The model under review builds one solid part; all positions refer to its coordinate system, in mm. A direction names the side the tool comes from. Give positions to 0.01 mm unless a question says otherwise; leave off trailing zeros. Order: outer loops, then holes, each group sorted by start corner. A loop starts at its lowest first (then second) coordinate and runs counter-clockwise, first axis right, second up. Notation, with made-up numbers: M 37.25,36 L 86.25,36 A15 cw 86.25,50 Z; hole C 79.25,32 d2. An arc over 180 degrees is marked long. One line per question, with ' | ' between items. Start each with the question number.
1. Wall thickness on L1, parallel to Y at x = 0, z = -8.95; L2, parallel to X at y = 5.25, z = 2; L3, parallel to X at y = 2.25, z = 5.75: over which ranges is each line inside the solid? List them lowest first.
2. For faces 1 (the face through (-2.2, -10, -9.5)), 2 (the face through (3, 3, 1)), 3 (the face through (0, -7, -8.5)), list the 3-axis set-ups (+Z, -Z, +X, -X, +Y, -Y) from which the entire face can be reached by the end or side of a thin tool; tool diameter is ignored.
3. We need section B-B on y = -10. Write out the cut boundary in (x, z).
4. Insertion check: P1, Ø3.5, axis at x = 0, y = -10, coming from the -Z side; P2, Ø1, axis at x = -0.5, y = -2, coming from the +Z side; P3, Ø8, axis at y = -9.5, z = -2, coming from the +X side; P4, Ø2.5, axis at x = -0.5, z = 7.5, coming from the -Y side. Each pin has a flat end and moves straight along its axis. Give the tip position at first contact, or say it passes through.
5. We need section A-A on x = 0. Write out the cut boundary in (y, z), then the cut area to 3 significant figures.
6. The part is to be moulded in two halves that separate along X. For faces 4 (the face through (0, 3, -2.5)), 5 (the face through (-5.18, -19.4, -10.48)), 6 (the face through (0, 0, -5)), 7 (the face through (-3, 3, 1)), say which applies: +X half, -X half, draft (parallel to the pull), parting line (faces both ways), or undercut.
7. We need section C-C on z = -6. Write out the cut boundary in (x, y), then the cut area to 3 significant figures.
8. We need section D-D on y = 3.75. Write out the cut boundary in (x, z), then the cut area to 3 significant figures.
```python
from build123d import *

# Parameters (mm, degrees)
SKETCH1_W                      = 11.5
SKETCH1_H                      = 25
BOSS_EXTRUDE1_DEPTH            = 8
CUT_EXTRUDE1_DEPTH             = 6
SKETCH3_W                      = 11.5
SKETCH3_H                      = 4
BOSS_EXTRUDE2_DEPTH            = 20
CBORE_FOR_M3_SHCS1_D           = 3.2
CBORE_FOR_M3_SHCS1_CBORE_D     = 6.6
CBORE_FOR_M3_SHCS1_CBORE_DEPTH = 3
FILLET1_R                      = 2
CHAMFER1_SIZE                  = 0.4
CHAMFER2_SIZE                  = 0.4


with BuildPart() as part:
    # Sketch1 → Boss-Extrude1 (new body)
    with BuildSketch(Plane(origin=(0, 0, 0), x_dir=(1, 0, 0), z_dir=(0, 1, 0))):
        Rectangle(SKETCH1_W, SKETCH1_H)
    extrude(amount=BOSS_EXTRUDE1_DEPTH)

    # Sketch2 → Cut-Extrude1 (cut)
    with BuildSketch(Plane.XZ):
        Polygon((-3, 12.5), (3, 12.5), (3, 11.5), (3.8, 11.5), (3.8, 4.5), (3, 4.5), (3, -2.5), (-3, -2.5), (-3, 4.5), (-3.8, 4.5), (-3.8, 11.5), (-3, 11.5), align=None)
    extrude(amount=-CUT_EXTRUDE1_DEPTH, mode=Mode.SUBTRACT)

    # Sketch3 → Boss-Extrude2 (add)
    with BuildSketch(Plane.XZ):
        with Locations((0, -10.5)):
            Rectangle(SKETCH3_W, SKETCH3_H)
    extrude(amount=BOSS_EXTRUDE2_DEPTH)

    # CBORE for M3 SHCS1 (through all)
    with Locations(Plane(origin=(0, 0, -12.5), x_dir=(-1, 0, 0), z_dir=(0, 0, -1))):
        with Locations((0, -10)):
            CounterBoreHole(CBORE_FOR_M3_SHCS1_D / 2, CBORE_FOR_M3_SHCS1_CBORE_D / 2, CBORE_FOR_M3_SHCS1_CBORE_DEPTH)

    # Fillet1
    fillet1_edges = [part.edges().sort_by_distance(p)[0] for p in [
        (-5.75, -20, -10.5),
        (5.75, -20, -10.5),
    ]]
    fillet(fillet1_edges, radius=FILLET1_R)

    # Chamfer1
    chamfer1_edges = [part.edges().sort_by_distance(p)[0] for p in [
        (5.75, 8, 0),
        (0, 8, -12.5),
        (-5.75, 8, 0),
        (0, 8, 12.5),
    ]]
    chamfer(chamfer1_edges, length=CHAMFER1_SIZE)

    # Chamfer2
    chamfer2_edges = [part.edges().sort_by_distance(p)[0] for p in [
        (4.375, 0, 12.5),
        (-3, 0, 12),
        (-3.4, 0, 11.5),
        (-3.8, 0, 8),
        (-3.4, 0, 4.5),
        (-3, 0, 1),
        (0, 0, -2.5),
        (3, 0, 1),
        (3.4, 0, 4.5),
        (3.8, 0, 8),
        (3.4, 0, 11.5),
        (3, 0, 12),
        (3, 3, 12.5),
        (0, 6, 12.5),
        (-3, 3, 12.5),
        (-5.75, 0, 2),
        (5.75, 0, 2),
        (-4.375, 0, 12.5),
        (3.3, -10, -12.5),
        (-1.6, -10, -9.5),
        (0, -20, -12.5),
        (0, -20, -8.5),
        (5.164213562, -19.414213562, -12.5),
        (-5.164213562, -19.414213562, -12.5),
        (-5.75, -9, -8.5),
        (5.75, -9, -8.5),
        (5.164213562, -19.414213562, -8.5),
        (-5.164213562, -19.414213562, -8.5),
        (-5.75, -5.2, -12.5),
        (5.75, -5.2, -12.5),
        (5.75, 3.8, 12.5),
        (-5.75, 3.8, 12.5),
    ]]
    chamfer(chamfer2_edges, length=CHAMFER2_SIZE)


solid = part.part
```
Entries:
1) L1: y = -20 to -11.6, -8.4 to 8 | L2: x = -5.75 to -3, 3 to 5.75 | L3: x = -5.75 to -3.8, 3.8 to 5.75
2) face 1: -Z | face 2: +Z, -Y | face 3: +Z, +X, -X, -Y
3) outline: M -5.75,-12.1 L -5.35,-12.5 L -3.7,-12.5 L -3.3,-12.1 L -3.3,-9.5 L -2,-9.5 L -1.6,-9.1 L -1.6,-8.5 L -5.35,-8.5 L -5.75,-8.9 Z; M 1.6,-9.1 L 2,-9.5 L 3.3,-9.5 L 3.3,-12.1 L 3.7,-12.5 L 5.35,-12.5 L 5.75,-12.1 L 5.75,-8.9 L 5.35,-8.5 L 1.6,-8.5 Z
4) P1: stops at z = -9.25 | P2: stops at z = -8.5 | P3: passes through | P4: stops at y = 6
5) outline: M -20,-12.1 L -19.6,-12.5 L -13.7,-12.5 L -13.3,-12.1 L -13.3,-9.5 L -12,-9.5 L -11.6,-9.1 L -11.6,-8.5 L -19.6,-8.5 L -20,-8.9 Z; M -8.4,-9.1 L -8,-9.5 L -6.7,-9.5 L -6.7,-12.1 L -6.3,-12.5 L 7.6,-12.5 L 8,-12.1 L 8,12.1 L 7.6,12.5 L 6.4,12.5 L 6,12.1 L 6,-2.5 L 0.4,-2.5 L 0,-2.9 L 0,-8.5 L -8.4,-8.5 Z | area: 166 mm^2
6) face 4: undercut | face 5: -X half | face 6: draft | face 7: undercut
7) outline: M -5.75,0.4 L -5.35,0 L 5.35,0 L 5.75,0.4 L 5.75,7.6 L 5.35,8 L -5.35,8 L -5.75,7.6 Z | area: 91.7 mm^2
8) outline: M -5.75,-12.1 L -5.35,-12.5 L 5.35,-12.5 L 5.75,-12.1 L 5.75,12.1 L 5.35,12.5 L 3.4,12.5 L 3,12.1 L 3,11.5 L 3.8,11.5 L 3.8,4.5 L 3,4.5 L 3,-2.5 L -3,-2.5 L -3,4.5 L -3.8,4.5 L -3.8,11.5 L -3,11.5 L -3,12.1 L -3.4,12.5 L -5.35,12.5 L -5.75,12.1 Z | area: 186 mm^2
